```python
from build123d import *

# Parameters (mm, degrees)
ESBO_O1_R                = 50
RESSALTO_EXTRUS_O2_DEPTH = 200
ESBO_O5_R                = 70
RESSALTO_EXTRUS_O3_DEPTH = 10
RESSALTO_EXTRUS_O4_START = 10
ESBO_O6_R                = 70
RESSALTO_EXTRUS_O4_DEPTH = 10
ESBO_O7_R                = 40
CORTE_EXTRUS_O3_DEPTH    = 220


with BuildPart() as part:
    # Esboço1 → Ressalto-extrusão2 (new body)
    with BuildSketch(Plane(origin=(0, 0, 0), x_dir=(1, 0, 0), z_dir=(0, 1, 0))):
        with Locations(Location((0, 0, 0), (0, 0, 270))):
            Circle(ESBO_O1_R)
    extrude(amount=RESSALTO_EXTRUS_O2_DEPTH)

    # Esboço5 → Ressalto-extrusão3 (add)
    with BuildSketch(Plane(origin=(0, 200, 0), x_dir=(1, 0, 0), z_dir=(0, 1, 0))):
        with Locations(Location((0, 0, 0), (0, 0, 270))):
            Circle(ESBO_O5_R)
    extrude(amount=RESSALTO_EXTRUS_O3_DEPTH)

    # Esboço6 → Ressalto-extrusão4 (add)
    with BuildSketch(Plane(origin=(0, 0, 0), x_dir=(-1, 0, 0), z_dir=(0, -1, 0)).offset(RESSALTO_EXTRUS_O4_START)):
        with Locations(Location((0, 0, 0), (0, 0, 270))):
            Circle(ESBO_O6_R)
    extrude(amount=-RESSALTO_EXTRUS_O4_DEPTH)

    # Esboço7 → Corte-extrusão3 (cut)
    with BuildSketch(Plane(origin=(0, -10, 0), x_dir=(-1, 0, 0), z_dir=(0, -1, 0))):
        with Locations(Location((0, 0, 0), (0, 0, 90))):
            Circle(ESBO_O7_R)
    extrude(amount=-CORTE_EXTRUS_O3_DEPTH, mode=Mode.SUBTRACT)


solid = part.part
```
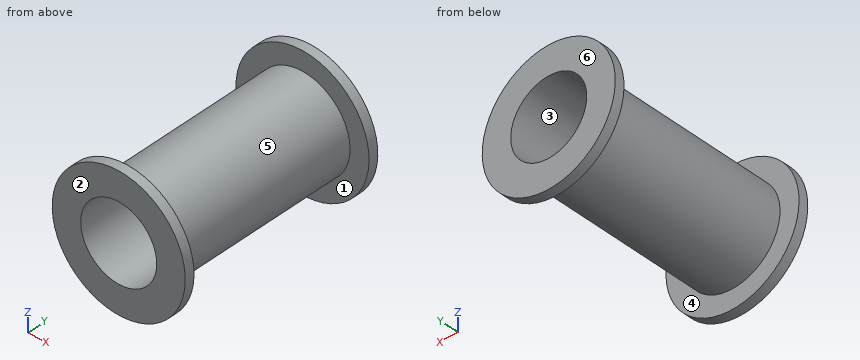
The listing builds one solid part. Answer for the finished solid, in the listing's coordinates (mm). Face numbers are marked on the shaded views. A direction names the side the tool comes from. Round coordinates to 2 decimals unless told otherwise and drop trailing zeros. Order: outer loops, then holes, each group sorted by start corner. A loop starts at its lowest first (then second) coordinate and runs counter-clockwise, first axis right, second up. Notation, with made-up numbers: (14, -10.5) - (61, -10.5) arc R23 ccw to (61, 9.5) - close; hole circle Ø6 at (-5, -35.75). An arc over 180 degrees is marked (long way). Put each result on its own line as item: value. Start each with the question number.
(1) Determine the mould class of the marked faces 3, 4, 5 and 6 for opening direction Y: released by +Y, released by -Y, zero draft, split by the parting line, or undercut.
(2) Find section B-B (z = 0). Give the vertices of the cut face in (x, y).
(3) For the marked faces 1 and 2, determine the directions among +Z, -Z, +X, -X, +Y, -Y from which every point of the face is accessible in a straight line to the end or side of a thin tool.
(4) Straight lines are drawn through the part: probe 1 along X at (y, z) = (119, 0); probe 2 along Y at (x, z) = (59.5, -29.5); probe 3 along Z at (x, y) = (2, 53). For each, find the intervals that lie inside material, in ascending order. Write a range as from..to.
(5) Find section C-C (y = 122.5). Give the vertices of the cut face in (x, z).
(6) Find section A-A (x = 0). Give the vertices of the cut face in (y, z).
(7) Find section D-D (z = 56.5). Give the vertices of the cut face in (x, y).
(8) Given P1, Ø1.5, axis at y = 131, z = -22.5, coming from the +X side; P2, Ø6, axis at y = 27, z = 35, coming from the +X side; P3, Ø10, axis at x = -27.5, y = 27.5, coming from the +Z side; P4, Ø6, axis at x = 51, z = -55, coming from the -Y side, each flat-ended and moving along its own axis, determine where each tip first touches the part or whether it passes through.
Reply:
1. face 3: zero draft
1. face 4: undercut
1. face 5: undercut
1. face 6: released by +Y
2. outline: (-70, -10) - (-40, -10) - (-40, 210) - (-70, 210) - (-70, 200) - (-50, 200) - (-50, 0) - (-70, 0) - close; (40, -10) - (70, -10) - (70, 0) - (50, 0) - (50, 200) - (70, 200) - (70, 210) - (40, 210) - close
3. face 1: none
3. face 2: +Z, -Z, +X, -X, -Y
4. probe 1: -50..-40, 40..50
4. probe 2: -10..0, 200..210
4. probe 3: -49.96..-39.95, 39.95..49.96
5. outline: circle Ø100 at (0, 0); hole circle Ø80 at (0, 0)
6. outline: (-10, -70) - (0, -70) - (0, -50) - (200, -50) - (200, -70) - (210, -70) - (210, -40) - (-10, -40) - close; (-10, 40) - (210, 40) - (210, 70) - (200, 70) - (200, 50) - (0, 50) - (0, 70) - (-10, 70) - close
7. outline: (-41.32, -10) - (41.32, -10) - (41.32, 0) - (-41.32, 0) - close; (-41.32, 200) - (41.32, 200) - (41.32, 210) - (-41.32, 210) - close
8. P1: x = 45.02
8. P2: x = 38.42
8. P3: z = 44.65
8. P4: through
